```python
from build123d import *

# Parameters (mm, degrees)
F1_DEPTH = 1270
F2_R     = 44.45
F3_DEPTH = 88.901
F4_R     = 54.0385
F5_DEPTH = 6.35
F6_SIZE  = 1.524
F7_SIZE  = 1.524


with BuildPart() as f1:
    # F0 (on Right) → F1 (new body, symmetric)
    with BuildSketch(Plane.YZ):
        Polygon((25.4, 0), (-25.4, 0), (-50.8, -9.244844), (-50.8, -88.9), (50.8, -88.9), (50.8, -9.244844), align=None)
    extrude(amount=F1_DEPTH, both=True)

    # F2 (on Top) → F3 (cut, through all)
    with BuildSketch(Plane.XY):
        with Locations((1143, 0)):
            Circle(F2_R)
        with Locations((-1143, 0)):
            Circle(F2_R)
    extrude(amount=-F3_DEPTH, mode=Mode.SUBTRACT)

    # F4 (on face) → F5 (cut)
    with BuildSketch(Plane(origin=(0, 0, -88.9), x_dir=(1, 0, 0), z_dir=(0, 0, -1))):
        with Locations((1143, 0)):
            Circle(F4_R)
        with Locations((-1143, 0)):
            Circle(F4_R)
    extrude(amount=-F5_DEPTH, mode=Mode.SUBTRACT)

    # F6
    f6_edges = [f1.edges().sort_by_distance(p)[0] for p in [
        (1098.55, 0, -82.55),
    ]]
    chamfer(f6_edges, length=F6_SIZE)

    # F7
    f7_edges = [f1.edges().sort_by_distance(p)[0] for p in [
        (-1187.45, 0, -82.55),
    ]]
    chamfer(f7_edges, length=F7_SIZE)


solid = f1.part
```
Could you check a few things on this model? Use its own coordinates, in mm. A direction names the side the tool comes from. Round coordinates to 2 decimals unless told otherwise and drop trailing zeros. Loops run counter-clockwise (first coordinate to the right, second up) from the corner with the lowest first, then second, coordinate; pieces in that order, holes last.
Q1. Please list where these lines run through material, in increasing order: L1, parallel to X at y = -1, z = -75.5; L2, parallel to Y at x = -1143, z = -64; L3, parallel to X at y = -3.5, z = -39.5.
Q2. I want a section at B-B (z = -41). Write out the boundary of the cut face in (x, y), and give its area (3 significant figures).
Q3. I want a section at C-C (x = 233). Write out the boundary of the cut face in (y, z), and give its area (3 significant figures).
Q4. For P1, Ø1, axis at x = -561, y = -13, coming from the +Z side, with a flat end and sliding along its axis, tell me the tip position at first contact or that it passes through.
Q5. On a 3-axis mill with a long thin cutter (end or side, diameter ignored), from which of +Z, -Z, +X, -X, +Y, -Y can I reach the whole of each face in a straight line? I mean faces 1 (the flat face through (-1270, -1, -44)), 2 (the flat face through (1134.7, -45.4, -82.55)). Say none if no direction works.
Q6. I want a section at A-A (y = 0). Write out the boundary of the cut face in (x, z).
Q7. Thinking about a two-plate mould opening in Y: for faces 3 (the flat face through (18, -50.8, -49)), 4 (the flat face through (-1227, -1, -88.9)), 5 (the cylindrical face through (-1187.407, 1.954, -39.946)), 6 (the flat face through (18, 50.8, -50)), which applies, pulls with the +Y half, pulls with the -Y half, needs draft (parallel to the pull), parting line crosses it, or undercut?
Answer below:
1. L1: x = -1270 to -1187.44, -1098.56 to 1098.56, 1187.44 to 1270
1. L2: y = -50.8 to -44.45, 44.45 to 50.8
1. L3: x = -1270 to -1187.31, -1098.69 to 1098.69, 1187.31 to 1270
2. outline: (-1270, -50.8) - (1270, -50.8) - (1270, 50.8) - (-1270, 50.8) - close; hole circle Ø88.9 at (-1143, 0); hole circle Ø88.9 at (1143, 0)
2. area: 246,000 mm2
3. outline: (-50.8, -88.9) - (50.8, -88.9) - (50.8, -9.24) - (25.4, 0) - (-25.4, 0) - (-50.8, -9.24) - close
3. area: 8,800 mm2
4. P1: stops at z = 0
5. face 1: +Z, -Z, -X, +Y, -Y
5. face 2: -Z
6. outline: (-1270, -88.9) - (-1197.04, -88.9) - (-1197.04, -82.55) - (-1188.97, -82.55) - (-1187.45, -81.03) - (-1187.45, 0) - (-1270, 0) - close; (-1098.55, -81.03) - (-1097.03, -82.55) - (-1088.96, -82.55) - (-1088.96, -88.9) - (1088.96, -88.9) - (1088.96, -82.55) - (1097.03, -82.55) - (1098.55, -81.03) - (1098.55, 0) - (-1098.55, 0) - close; (1187.45, -81.03) - (1188.97, -82.55) - (1197.04, -82.55) - (1197.04, -88.9) - (1270, -88.9) - (1270, 0) - (1187.45, 0) - close
7. face 3: pulls with the -Y half
7. face 4: needs draft
7. face 5: undercut
7. face 6: pulls with the +Y half
